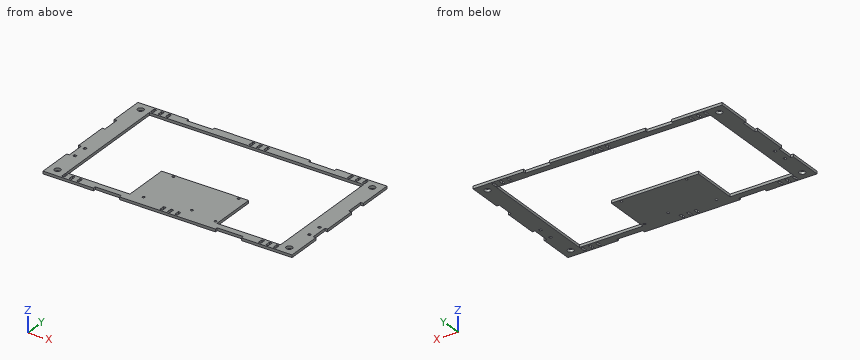
from build123d import *

# Parameters (mm, degrees)
F0_W     = 3
F0_H     = 6
F0_R     = 3.5
F0_R_2   = 1.375
F0_H_2   = 3
F1_DEPTH = 1.5


with BuildPart() as f1:
    # F0 (on Top) → F1 (new body, symmetric)
    with BuildSketch(Plane.XY):
        Polygon((-85, 80), (-143, 80), (-143, 40), (-140, 40), (-140, 20), (-143, 20), (-143, -20), (-140, -20), (-140, -40), (-143, -40), (-143, -80), (-85, -80), (-85, -77), (-55, -77), (-55, -80), (55, -80), (55, -77), (85, -77), (85, -80), (143, -80), (143, -40), (140, -40), (140, -20), (143, -20), (143, 20), (140, 20), (140, 40), (143, 40), (143, 80), (85, 80), (85, 77), (55, 77), (55, 80), (-55, 80), (-55, 77), (-85, 77), align=None)
        with Locations((-121.5, -75)):
            Rectangle(F0_W, F0_H, mode=Mode.SUBTRACT)
        with Locations((-113, -75)):
            Rectangle(F0_W, F0_H, mode=Mode.SUBTRACT)
        with Locations((-133, -70)):
            Circle(F0_R, mode=Mode.SUBTRACT)
        with Locations((-104.5, -75)):
            Rectangle(F0_W, F0_H, mode=Mode.SUBTRACT)
        with Locations((-36.03, -67.46)):
            Circle(F0_R_2, mode=Mode.SUBTRACT)
        Polygon((-7, -75), (-7, -78), (-10, -78), (-10, -75), (-10, -72), (-7, -72), align=None, mode=Mode.SUBTRACT)
        with Locations((-134.681027, -38.5)):
            Rectangle(F0_W, F0_H_2, mode=Mode.SUBTRACT)
        with Locations((-134.681027, -21.5)):
            Rectangle(F0_W, F0_H_2, mode=Mode.SUBTRACT)
        with Locations((-34.762099, -19.2)):
            Circle(F0_R_2, mode=Mode.SUBTRACT)
        Polygon((1.5, -78), (0, -78), (-1.5, -78), (-1.5, -75), (-1.5, -72), (1.5, -72), (1.5, -75), align=None, mode=Mode.SUBTRACT)
        with Locations((8.5, -75)):
            Rectangle(F0_W, F0_H, mode=Mode.SUBTRACT)
        with Locations((16.04, -62.38)):
            Circle(F0_R_2, mode=Mode.SUBTRACT)
        with Locations((46.52, -67.46)):
            Circle(F0_R_2, mode=Mode.SUBTRACT)
        with Locations((104.5, -75)):
            Rectangle(F0_W, F0_H, mode=Mode.SUBTRACT)
        with Locations((113, -75)):
            Rectangle(F0_W, F0_H, mode=Mode.SUBTRACT)
        with Locations((121.5, -75)):
            Rectangle(F0_W, F0_H, mode=Mode.SUBTRACT)
        with Locations((133, -70)):
            Circle(F0_R, mode=Mode.SUBTRACT)
        with Locations((40.17, -19.2)):
            Circle(F0_R_2, mode=Mode.SUBTRACT)
        with Locations((134.681027, -38.5)):
            Rectangle(F0_W, F0_H_2, mode=Mode.SUBTRACT)
        with Locations((134.681027, -21.5)):
            Rectangle(F0_W, F0_H_2, mode=Mode.SUBTRACT)
        with Locations((-133, 70)):
            Circle(F0_R, mode=Mode.SUBTRACT)
        with Locations((-121.5, 75)):
            Rectangle(F0_W, F0_H, mode=Mode.SUBTRACT)
        with Locations((-113, 75)):
            Rectangle(F0_W, F0_H, mode=Mode.SUBTRACT)
        with Locations((-104.5, 75)):
            Rectangle(F0_W, F0_H, mode=Mode.SUBTRACT)
        Polygon((-10, 78), (-7, 78), (-7, 75), (-7, 72), (-10, 72), (-10, 75), align=None, mode=Mode.SUBTRACT)
        Polygon((-123, 70), (123, 70), (123, -70), (50, -70), (50, -16.66), (-43, -16.66), (-50, -16.66), (-50, -70), (-123, -70), align=None, mode=Mode.SUBTRACT)
        Polygon((1.5, 75), (1.5, 72), (-1.5, 72), (-1.5, 75), (-1.5, 78), (0, 78), (1.5, 78), align=None, mode=Mode.SUBTRACT)
        with Locations((8.5, 75)):
            Rectangle(F0_W, F0_H, mode=Mode.SUBTRACT)
        with Locations((104.5, 75)):
            Rectangle(F0_W, F0_H, mode=Mode.SUBTRACT)
        with Locations((113, 75)):
            Rectangle(F0_W, F0_H, mode=Mode.SUBTRACT)
        with Locations((121.5, 75)):
            Rectangle(F0_W, F0_H, mode=Mode.SUBTRACT)
        with Locations((133, 70)):
            Circle(F0_R, mode=Mode.SUBTRACT)
    extrude(amount=F1_DEPTH, both=True)


solid = f1.part
Could you check a few things on this model? Use its own coordinates, in mm. Give positions to 0.01 mm unless a question says otherwise; leave off trailing zeros. Write each loop counter-clockwise with the first axis right and the second up, starting at its lowest first coordinate (ties: lowest second). Pieces come first, ordered by that corner, then holes. Notation, with made-up numbers: (-32.5, 25.25) - (12.5, 25.25) arc R23 cw to (12.5, 36.25) - close; hole circle Ø4 at (3, -28). An arc over 180 degrees is marked (long way). Use CSV: the item, a comma, the result in double quotes. Start each with the question number.
Item 1: I want a section at B-B, the plane y = 15. Please give me the cut outline in (x, z), then the cut area to 3 significant figures.
Item 2: I'm going to push flat-ended pins straight in: pin 1 (1.5 mm diameter, centred on x = 66.5, z = 0.5, fed in from +Y); pin 2 (3 mm diameter, centred on x = 40.17, y = -19.2, fed in from +Z); pin 3 (1.6 mm diameter, centred on x = -34.76, y = -19.2, fed in from -Z); pin 4 (1 mm diameter, centred on y = -23.5, z = 1, fed in from +X). Where does each tip first touch, or does it pass through?
Item 3: I want a section at D-D, the plane z = -0.3. Give the number of separate pieces and of enclosed holes in the cut face, then the cut area to 3 significant figures.
Item 4: If I drill on line 1 along Y through (x, z) = (133, -0.5); line 2 along Y through (x, z) = (-120.5, 0.5); line 3 along Y through (x, z) = (-10.5, 1.25), over which ranges is the centre line in solid material (lowest first)?
Item 5: I want a section at C-C, the plane y = -54.5. Please give me the cut outline in (x, z).
Item 6: I want a section at A-A, the plane x = -24.5. Please give me the cut outline in (y, z), then the cut area to 3 significant figures.
Findings:
1,outline,"(-143, -1.5) - (-123, -1.5) - (-123, 1.5) - (-143, 1.5) - close; (123, -1.5) - (143, -1.5) - (143, 1.5) - (123, 1.5) - close"
1,area,"120 mm2"
2,pin 1,"stops at y = 77"
2,pin 2,"stops at z = 1.5"
2,pin 3,"passes through"
2,pin 4,"stops at x = 140"
3,separate pieces,"1"
3,enclosed holes,"32"
3,area,"15,500 mm2"
4,line 1,"y = -80 to -73.5, -66.5 to 66.5, 73.5 to 80"
4,line 2,"y = -80 to -78, -72 to -70, 70 to 72, 78 to 80"
4,line 3,"y = -80 to -16.66, 70 to 80"
5,outline,"(-143, -1.5) - (-123, -1.5) - (-123, 1.5) - (-143, 1.5) - close; (-50, -1.5) - (50, -1.5) - (50, 1.5) - (-50, 1.5) - close; (123, -1.5) - (143, -1.5) - (143, 1.5) - (123, 1.5) - close"
6,outline,"(-80, -1.5) - (-16.66, -1.5) - (-16.66, 1.5) - (-80, 1.5) - close; (70, -1.5) - (80, -1.5) - (80, 1.5) - (70, 1.5) - close"
6,area,"220 mm2"
